Geometry: see drawing. Coordinates: mm, zero at the bounding-box minimum. Give positions to 0.01 mm unless a question says otherwise; leave off trailing zeros. Order: outer loops, then holes, each group sorted by start corner. A loop starts at its lowest first (then second) coordinate and runs counter-clockwise, first axis right, second up. Notation, with made-up numbers: M -34,2.5 L -10,2.5 A21 ccw -10,40.5 Z; hole C 68,11.25 d11. An arc over 180 degrees is marked long. Answer as a JSON object with one key per item and string values. Group by question number.
1. Pull-direction query (X, two-part tool) for the marked faces 1, 2 and 3; classes: +X half, -X half, draft (parallel to the pull), parting line (faces both ways), or undercut.
2. Pin query (flat end, axial travel): P1, Ø1, axis at x = 46, z = 1.5, coming from the +Y side; P2, Ø4.5, axis at x = 10, y = 35, coming from the -Z side; P3, Ø1, axis at x = 56, z = 3, coming from the -Y side. Return the tip coordinate at first contact, or that it passes through.
3. Section query D-D (x = 60). Output: boundary loops of the cut face in (y, z).
4. Section query C-C (z = 0.8). Output: boundary loops of the cut face in (x, y).
5. Section query A-A (x = 35). Output: boundary loops of the cut face in (y, z), plus the area to 4 significant figures.
6. Material intervals for L1, parallel to Y at x = 35, z = 1.1; L2, parallel to Y at x = 61, z = 2.8; L3, parallel to X at y = 40.5, z = 2.4, sorted ascending. Write a range as [from, to].
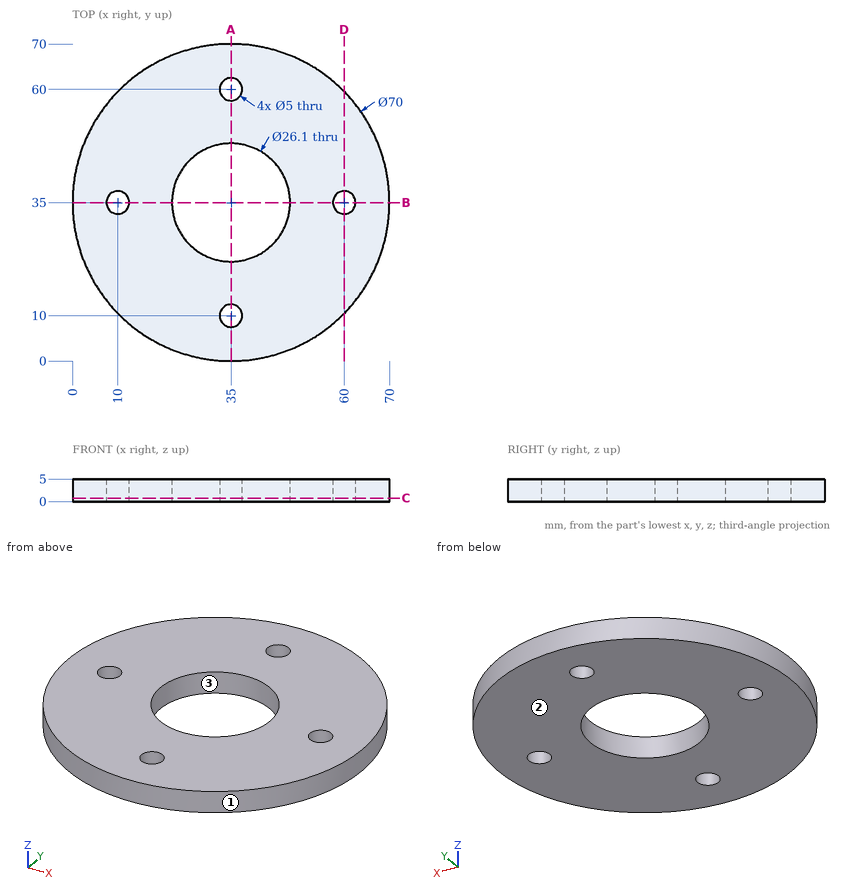
Answer sheet:
{
 "1": {"face 1": "parting line", "face 2": "draft", "face 3": "undercut"},
 "2": {"P1": "y = 68.39", "P2": "through", "P3": "y = 6.63"},
 "3": {"outline": "M 10.51,0 L 32.5,0 L 32.5,5 L 10.51,5 Z; M 37.5,0 L 59.49,0 L 59.49,5 L 37.5,5 Z"},
 "4": {"outline": "C 35,35 d70; hole C 10,35 d5; hole C 35,35 d26.1; hole C 35,10 d5; hole C 35,60 d5; hole C 60,35 d5"},
 "5": {"outline": "M 0,0 L 7.5,0 L 7.5,5 L 0,5 Z; M 12.5,0 L 21.95,0 L 21.95,5 L 12.5,5 Z; M 48.05,0 L 57.5,0 L 57.5,5 L 48.05,5 Z; M 62.5,0 L 70,0 L 70,5 L 62.5,5 Z", "area": "169.5 mm^2"},
 "6": {"L1": "[0, 7.5], [12.5, 21.95], [48.05, 57.5], [62.5, 70]", "L2": "[11.57, 32.71], [37.29, 58.43]", "L3": "[0.43, 23.17], [46.83, 69.57]"}
}
